```python
from build123d import *

# Parameters (mm, degrees)
SKETCH_4_R               = 4
CUT_EXTRUDE_1_DEPTH      = 2
PATTERN_CIRCULAR_1_COUNT = 6
CHAMFER_1_SIZE           = 0.6


with BuildPart() as part:
    # Эскиз1 → Повернуть1 (revolve)
    with BuildSketch(Plane.XY):
        Polygon((0, 0), (-37.5, 0), (-37.5, -2.5), (-24.65, -2.5), (-24.65, -5.5), (-20, -5.5), (-20, -2.5), (0, -2.5), align=None)
    revolve(axis=Axis((0, 0, 0), (0, 1, 0)))

    # Эскиз4 → Cut-Extrude 1 (cut)
    with BuildSketch(Plane.XZ.offset(2.5)):
        with Locations((-31, 0)):
            Circle(SKETCH_4_R)
    cut_extrude_1 = extrude(amount=-CUT_EXTRUDE_1_DEPTH, mode=Mode.SUBTRACT)

    # Круговой массив1: Cut-Extrude 1 ×6 about axis
    pattern_circular_1_axis = Axis((0, 0, 0), (0, 1, 0))
    for i in range(1, PATTERN_CIRCULAR_1_COUNT):
        add(cut_extrude_1.rotate(pattern_circular_1_axis, i * 360 / PATTERN_CIRCULAR_1_COUNT), mode=Mode.SUBTRACT)

    # Фаска1
    chamfer_1_edges = [part.edges().sort_by_distance(p)[0] for p in [
        (24.65, -5.5, 0),
        (37.5, 0, 0),
    ]]
    chamfer(chamfer_1_edges, length=CHAMFER_1_SIZE)


solid = part.part
```
Verification items for the finished model (mm, model axes). A direction names the side the tool comes from. Give positions to 0.01 mm unless a question says otherwise; leave off trailing zeros. Loops run counter-clockwise (first coordinate to the right, second up) from the corner with the lowest first, then second, coordinate; pieces in that order, holes last. Notation, with made-up numbers: M 43.25,8 L 59.25,8 A7 ccw 59.25,14 Z; hole C 74,78.5 d9. An arc over 180 degrees is marked long. One line per question, with ' | ' between items.
Item 1: Section check A-A, the plane y = -4. Record the cut outline in (x, z), plus the area to 3 significant figures.
Completed:
outline: C 0,0 d49.3; hole C 0,0 d40 | area: 652 mm^2
Item 2: Tool access check on faces 5 (the face through (-34.2, -1.5, -2.4)), 6 (the face through (-1, 0, 1)). Record the directions out of +Z, -Z, +X, -X, +Y, -Y that give a thin tool (end or side, any length) a straight path to the whole face; none if there is none.
Completed:
face 5: -Y | face 6: +Z, -Z, +X, -X, +Y
Item 3: Section check B-B, the plane z = 0. Record the cut outline in (x, y), plus the area to 3 significant figures.
Completed:
outline: M -37.5,-2.5 L -35,-2.5 L -35,-0.5 L -27,-0.5 L -27,-2.5 L -24.65,-2.5 L -24.65,-4.9 L -24.05,-5.5 L -20,-5.5 L -20,-2.5 L 20,-2.5 L 20,-5.5 L 24.05,-5.5 L 24.65,-4.9 L 24.65,-2.5 L 27,-2.5 L 27,-0.5 L 35,-0.5 L 35,-2.5 L 37.5,-2.5 L 37.5,-0.6 L 36.9,0 L -36.9,0 L -37.5,-0.6 Z | area: 183 mm^2
Item 4: Thickness scan on line 1 (Z direction, x = 0, y = -3.65); line 2 (X direction, y = -1.15, z = 30.5); line 3 (Z direction, x = -15.5, y = -2.05). Record the ranges inside material, lowest first. Write a range as [from, to].
Completed:
line 1: z = [-24.65, -20], [20, 24.65] | line 2: x = [-21.82, -17.13], [-13.87, 13.87], [17.13, 21.82] | line 3: z = [-34.15, -30.85], [-22.85, 22.85], [30.85, 34.15]
Item 5: Draft check along X on faces 1 (the face through (16, -0.5, 27)), 2 (the face through (4.88, -1.56, 37.18)), 3 (the face through (0, -2.5, 0)), 4 (the face through (-8, -2.5, -24)). Enter one of: +X half, -X half, draft (parallel to the pull), parting line (faces both ways), or undercut.
Completed:
face 1: undercut | face 2: parting line | face 3: undercut | face 4: draft
Item 6: Depth check by flat-ended pin: P1, Ø9, axis at x = 17, z = 25.5, coming from the -Y side; P2, Ø3, axis at y = -3.5, z = 14, coming from the +X side; P3, Ø2.5, axis at x = 29.5, z = 0.5, coming from the -Y side. Enter the tip coordinate at first touch or a pass-through.
Completed:
P1: stops at y = -2.5 | P2: stops at x = 35.22 | P3: stops at y = -0.5
